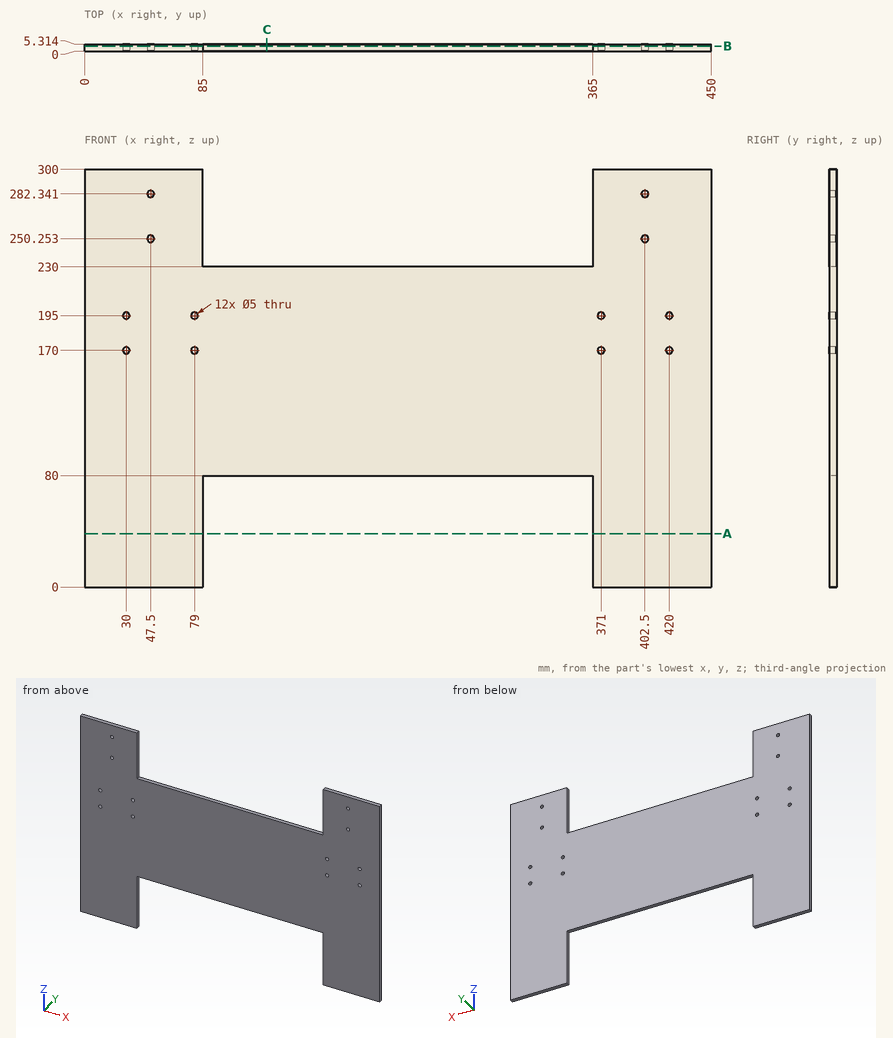
Study the drawing (mm; zero at the part's minimum x, y, z) and answer. Give positions to 0.01 mm unless a question says otherwise; leave off trailing zeros. Write each loop counter-clockwise with the first axis right and the second up, starting at its lowest first coordinate (ties: lowest second). Pieces come first, ordered by that corner, then holes. Notation, with made-up numbers: (64.25, 14.25) -> (120.25, 14.25) arc R20 ccw to (120.25, 37.25) -> close; hole circle Ø1 at (42.25, 63.5). An arc over 180 degrees is marked (long way). Write item = value, one per line. Start each with the question number.
1) The part is cut by section C-C, the plane x = 131. Determine the outline of the cut face in (y, z).
2) The part is cut by section A-A, the plane z = 38.5. Determine the outline of the cut face in (x, y).
3) Straight lines are drawn through the part: line 1 along X through (y, z) = (3.4, 170); line 2 along Z through (x, y) = (79, 2.7); line 3 along Z through (x, y) = (47.5, 4.15). For each, find the intervals that lie inside material, in ascending order.
4) Each of these flat-tipped pins is pushed along its axis until it touches: pin 1 (6.5 mm diameter, centred on x = 79, z = 195, fed in from -Y); pin 2 (3 mm diameter, centred on x = 294.5, y = 3.5, fed in from -Z). Where does it stop, or does it pass through?
5) The part is cut by section B-B, the plane y = 3.8. Count the separate pieces of the cut face and the enclosed holes in it, and give its area (3 significant figures).
Solutions:
q1.outline = (0, 80) -> (5.31, 80) -> (5.31, 230) -> (0, 230) -> close
q2.outline = (0, 0) -> (85, 0) -> (85, 5.31) -> (0, 5.31) -> close; (365, 0) -> (450, 0) -> (450, 5.31) -> (365, 5.31) -> close
q3.line_1 = 0 to 27.5, 32.5 to 76.5, 81.5 to 368.5, 373.5 to 417.5, 422.5 to 450
q3.line_2 = 0 to 167.5, 172.5 to 192.5, 197.5 to 300
q3.line_3 = 0 to 247.75, 252.75 to 279.84, 284.84 to 300
q4.pin_1 = 0
q4.pin_2 = 80
q5.separate_pieces = 1
q5.enclosed_holes = 12
q5.area = 92,800 mm²
